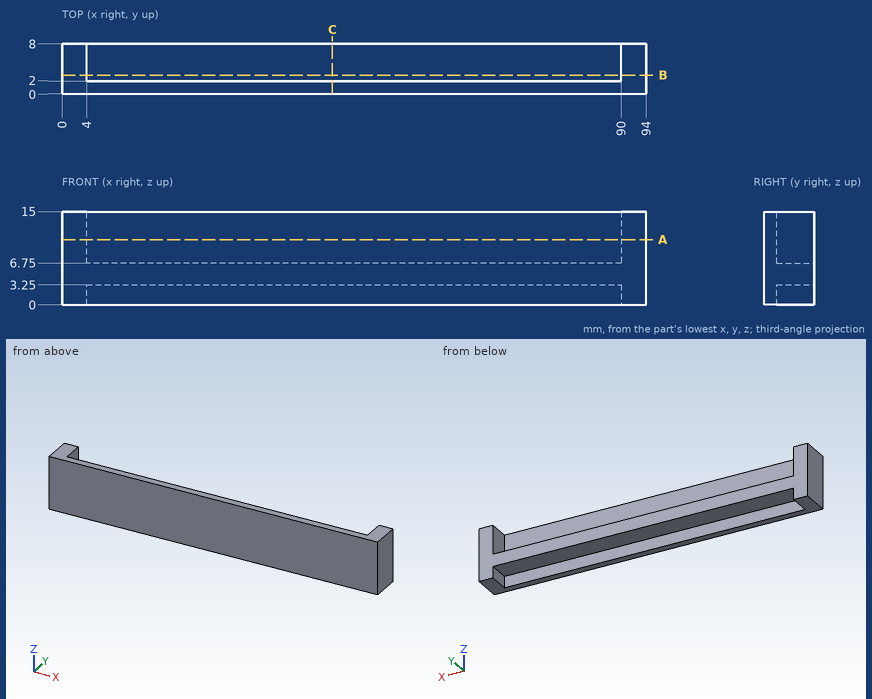
Could you check a few things on this drawing? It's one solid part, dimensions in mm from its lowest x, y, z. Coordinates: 2 decimals unless noted, no trailing zeros. Write each loop counter-clockwise with the first axis right and the second up, starting at its lowest first coordinate (ties: lowest second). Pieces come first, ordered by that corner, then holes. Notation, with made-up numbers: M 32,6 L 83,6 A31 ccw 83,38 Z; hole C 5,79.5 d7. An arc over 180 degrees is marked long. One line per question, with ' | ' between items.
1) Imagine slicing it at A-A, the plane z = 10.5. Write out the boundary of the cut face in (x, y).
Checks:
outline: M 0,0 L 94,0 L 94,8 L 90,8 L 90,2 L 4,2 L 4,8 L 0,8 Z
2) Imagine slicing it at B-B, the plane y = 3. Write out the boundary of the cut face in (x, z).
Checks:
outline: M 0,0 L 4,0 L 4,3.25 L 90,3.25 L 90,0 L 94,0 L 94,15 L 90,15 L 90,6.75 L 4,6.75 L 4,15 L 0,15 Z
3) Imagine slicing it at C-C, the plane x = 43.5. Write out the boundary of the cut face in (y, z), and give its area (3 significant figures).
Checks:
outline: M 0,0 L 2,0 L 2,3.25 L 8,3.25 L 8,6.75 L 2,6.75 L 2,15 L 0,15 Z | area: 51.0 mm²
4) For pin 1 Ø4 at (x, y) = (30, 5.5) entering from +Z; pin 2 Ø1.6 at (x, z) = (30, 1) entering from +Y, each with a flat end and sliding along its axis, tell me the tip position at first contact or that it passes through.
Checks:
pin 1: z = 6.75 | pin 2: y = 2
5) I need wall thicknesses on probe 1 along X at (y, z) = (4, 11); probe 2 along Z at (x, y) = (44, 3.75); probe 3 along Y at (x, z) = (54, 14). Which ranges of each line are inside material? Lowest first, please. Write a range as [from, to].
Checks:
probe 1: [0, 4], [90, 94] | probe 2: [3.25, 6.75] | probe 3: [0, 2]
